Model file for the job. Use its own axes, mm. A direction names the side the tool comes from. Round coordinates to 2 decimals unless told otherwise and drop trailing zeros. Loops run counter-clockwise (first coordinate to the right, second up) from the corner with the lowest first, then second, coordinate; pieces in that order, holes last. Notation, with made-up numbers: (-26, 63.5) - (-4, 63.5) arc R23 ccw to (-4, 75.5) - close; hole circle Ø4 at (48.25, 14.5). An arc over 180 degrees is marked (long way). Use one line per item in the form item = value.
from build123d import *

# Parameters (mm, degrees)
F0_W     = 63.3
F0_H     = 58
F1_DEPTH = 15
F2_W     = 60.7
F2_H     = 54.9
F3_DEPTH = 13
F4_R     = 1.5
F5_DEPTH = 15.001


with BuildPart() as f1:
    # F0 (on Top) → F1 (new body)
    with BuildSketch(Plane.XY):
        Rectangle(F0_W, F0_H)
    extrude(amount=F1_DEPTH)

    # F2 (on face) → F3 (cut)
    with BuildSketch(Plane.XY.offset(15)):
        Rectangle(F2_W, F2_H)
    extrude(amount=-F3_DEPTH, mode=Mode.SUBTRACT)

    # F4 (on face) → F5 (cut, through all)
    with BuildSketch(Plane(origin=(0, 0, 0), x_dir=(1, 0, 0), z_dir=(0, 0, -1))):
        with Locations((28.8, 0)):
            Circle(F4_R)
        with Locations((-28.8, 0)):
            Circle(F4_R)
    extrude(amount=-F5_DEPTH, mode=Mode.SUBTRACT)


solid = f1.part
1. Cut at D-D, the plane x = -22. Give the cut face in (y, z).
Geometry check:
outline = (-29, 0) - (29, 0) - (29, 15) - (27.45, 15) - (27.45, 2) - (-27.45, 2) - (-27.45, 15) - (-29, 15) - close
2. Cut at C-C, the plane z = 6.75. Give the cut face in (x, y), plus the area to 3 significant figures.
Geometry check:
outline = (-31.65, -29) - (31.65, -29) - (31.65, 29) - (-31.65, 29) - close; hole (-30.35, -27.45) - (30.35, -27.45) - (30.35, 27.45) - (-30.35, 27.45) - close
area = 339 mm^2
3. Flat gauge pins, fed straight in: pin 1 (1.5 mm diameter, centred on x = -8.5, y = 5.5, fed in from +Z); pin 2 (4 mm diameter, centred on x = -28.8, y = 0, fed in from +Z); pin 3 (2.5 mm diameter, centred on x = 28.8, y = 0, fed in from -Z). Where does each tip first touch, or does it go through?
Geometry check:
pin_1 = 2
pin_2 = 15
pin_3 = through
4. Cut at B-B, the plane y = 0. Give the cut face in (x, z), plus the area to 3 significant figures.
Geometry check:
outline = (-31.65, 0) - (-30.3, 0) - (-30.3, 2) - (-30.35, 2) - (-30.35, 15) - (-31.65, 15) - close; (-27.3, 0) - (27.3, 0) - (27.3, 2) - (-27.3, 2) - close; (30.3, 0) - (31.65, 0) - (31.65, 15) - (30.35, 15) - (30.35, 2) - (30.3, 2) - close
area = 148 mm^2
5. Tool access for faces 4 (the flat face through (31.65, 0, 7)), 5 (the flat face through (-30.35, 0, 9)): list every direction of +Z, -Z, +X, -X, +Y, -Y with a clear straight run to the whole face (end or side of a thin tool).
Geometry check:
face_4 = +Z, -Z, +X, +Y, -Y
face_5 = +Z
6. Wall check: probe 1 along X at (y, z) = (0, 1.3); probe 2 along Y at (x, z) = (-8, 7.5); probe 3 along Y at (x, z) = (28.8, 1.05). Give the ranges that are in metal, low to high.
Geometry check:
probe_1 = -31.65 to -30.3, -27.3 to 27.3, 30.3 to 31.65
probe_2 = -29 to -27.45, 27.45 to 29
probe_3 = -29 to -1.5, 1.5 to 29
7. Pull direction Y, two halves, no side cores. Call faces 1 (the flat face through (0, -29, 7)), 2 (the flat face through (0, 29, 7)), 3 (the flat face through (0, 27.45, 9)): +Y half, -Y half, draft (parallel to the pull), parting line (faces both ways), or undercut.
Geometry check:
face_1 = -Y half
face_2 = +Y half
face_3 = undercut
8. Cut at A-A, the plane x = 28.8. Give the cut face in (y, z).
Geometry check:
outline = (-29, 0) - (-1.5, 0) - (-1.5, 2) - (-27.45, 2) - (-27.45, 15) - (-29, 15) - close; (1.5, 0) - (29, 0) - (29, 15) - (27.45, 15) - (27.45, 2) - (1.5, 2) - close
